from build123d import *

# Parameters (mm, degrees)
SKETCH1_W           = 127
SKETCH1_H           = 12.7
SKETCH1_R           = 2.032
BOSS_EXTRUDE1_DEPTH = 3.175
BOSS_EXTRUDE2_DEPTH = 3.175


with BuildPart() as part:
    # Sketch1 → Boss-Extrude1 (new body)
    with BuildSketch(Plane.XY):
        Rectangle(SKETCH1_W, SKETCH1_H)
        with Locations((-57.15, 0)):
            Circle(SKETCH1_R, mode=Mode.SUBTRACT)
        with Locations((-38.1, 0)):
            Circle(SKETCH1_R, mode=Mode.SUBTRACT)
    extrude(amount=BOSS_EXTRUDE1_DEPTH)

    # Sketch2 → Boss-Extrude2 (add)
    with BuildSketch(Plane.XY.offset(3.175)):
        with BuildLine():
            Line((63.5, 6.35), (50.8, 6.35))
            ThreePointArc((50.8, 6.35), (57.15, 12.7), (63.5, 6.35))
        make_face()
    extrude(amount=-BOSS_EXTRUDE2_DEPTH)


solid = part.part
Work out the finished part from the listing and answer in its coordinate system (mm). A direction names the side the tool comes from. Coordinates: 2 decimals unless noted, no trailing zeros. Loops run counter-clockwise (first coordinate to the right, second up) from the corner with the lowest first, then second, coordinate; pieces in that order, holes last. Notation, with made-up numbers: (19.5, 32.25) -> (32.5, 32.25) arc R21 ccw to (32.5, 51.25) -> close; hole circle Ø11 at (46.5, -16.75). An arc over 180 degrees is marked (long way). Write each question's results on one line, items separated by ' | '. Start each with the question number.
1) For faces 4 (the flat face through (1, 1, 3.175)), 5 (the flat face through (-7, 6.35, 2)), determine the directions among +Z, -Z, +X, -X, +Y, -Y from which every point of the face is accessible in a straight line to the end or side of a thin tool.
2) Find section D-D on x = 26. Determine the outline of the cut face in (y, z) (3 decimals).
3) The mould has two halves that part along X. Classify faces 1 (the flat face through (-63.5, 0, 2)), 2 (the cylindrical face through (-40.13, 0.09, 1.57)), 3 (the cylindrical face through (57, 12.7, 1.6)): pulls with the +X half, pulls with the -X half, needs draft (parallel to the pull), parting line crosses it, or undercut.
4) Find section A-A on x = -38.1. Determine the outline of the cut face in (y, z) (3 decimals).
5) A flat-ended cylindrical pin translates along its axis: P1, Ø1.5, axis at y = 10, z = 2, coming from the -X side. Find the tip coordinate at first contact, or state that the pin passes through.
6) Consider line 1 along Y through (x, z) = (-57.15, 1.2); line 2 along Y through (x, z) = (-19.5, 0.65); line 3 along X through (y, z) = (12, 0.1). Determine where each line is inside the solid, lowest interval first.
7) Find section B-B on y = 0. Determine the outline of the cut face in (x, z) (3 decimals), then the cut area to 3 significant figures.
8) Find section C-C on z = 2.5. Determine the outline of the cut face in (x, y), then the cut area to 3 significant figures.
Response values:
1) face 4: +Z, +X, -X, +Y, -Y | face 5: +Z, -Z, -X, +Y
2) outline: (-6.35, 0) -> (6.35, 0) -> (6.35, 3.175) -> (-6.35, 3.175) -> close
3) face 1: pulls with the -X half | face 2: undercut | face 3: parting line crosses it
4) outline: (-6.35, 0) -> (-2.032, 0) -> (-2.032, 3.175) -> (-6.35, 3.175) -> close; (2.032, 0) -> (6.35, 0) -> (6.35, 3.175) -> (2.032, 3.175) -> close
5) P1: stops at x = 51.5
6) line 1: y = -6.35 to -2.03, 2.03 to 6.35 | line 2: y = -6.35 to 6.35 | line 3: x = 54.25 to 60.05
7) outline: (-63.5, 0) -> (-59.182, 0) -> (-59.182, 3.175) -> (-63.5, 3.175) -> close; (-55.118, 0) -> (-40.132, 0) -> (-40.132, 3.175) -> (-55.118, 3.175) -> close; (-36.068, 0) -> (63.5, 0) -> (63.5, 3.175) -> (-36.068, 3.175) -> close | area: 377 mm^2
8) outline: (-63.5, -6.35) -> (63.5, -6.35) -> (63.5, 6.35) arc R6.35 ccw to (50.8, 6.35) -> (-63.5, 6.35) -> close; hole circle Ø4.06 at (-57.15, 0); hole circle Ø4.06 at (-38.1, 0) | area: 1,650 mm^2
